CAD build for the part. Positions are in the model's coordinates, mm. Face numbers are marked on the shaded views. A direction names the side the tool comes from. Round coordinates to 2 decimals unless told otherwise and drop trailing zeros. Loops run counter-clockwise (first coordinate to the right, second up) from the corner with the lowest first, then second, coordinate; pieces in that order, holes last. Notation, with made-up numbers: M 33.5,86.5 L 62.5,86.5 A20 ccw 62.5,125.5 Z; hole C -8,-9.5 d9. An arc over 180 degrees is marked long. One line per item, written item: value. Start each with the question number.
from build123d import *


with BuildPart() as part:
    # Sketch1 → Revolve1 (revolve)
    with BuildSketch(Plane.XY):
        Polygon((0, 0), (-7.9629, 0), (-7.9629, -3.81), (-5.842, -5.334), (-5.842, -7.239), (-7.9629, -8.001), (-7.9629, -40.259), (-6.3754, -40.259), (-6.3754, -45.593), (-12.5, -45.593), (-12.5, -63.119), (-6.3754, -63.119), (-6.3754, -69.142247751), (-2.410616984, -74.041), (0, -74.041), align=None)
    revolve(axis=Axis((0, 0, 0), (0, 1, 0)))


solid = part.part
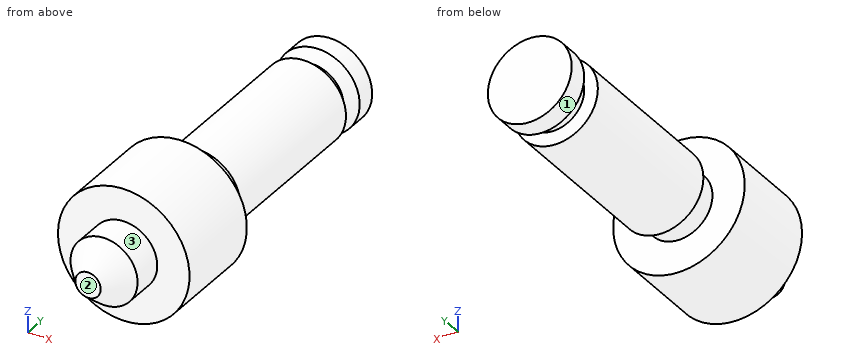
(1) Which spindle directions (+Z, -Z, +X, -X, +Y, -Y) get a long thin tool onto all of the face, cutting with end or side? Do the marked faces 1, 2 and 3. Say none if no direction does.
(2) Probe L1, parallel to Y at x = -6, z = -4; L2, parallel to Y at x = -2, z = -8.25; L3, parallel to Y at x = 6, z = 0.5. List the from-to ranges inside material, lowest first.
(3) Flat gauge pins, fed straight in: P1, Ø12, axis at x = 2.5, z = -8, coming from the -Y side; P2, Ø10, axis at x = 8, y = -17.5, coming from the -Z side; P3, Ø3, axis at x = -5.5, y = -60, coming from the +Z side; P4, Ø12, axis at x = -7, y = -8.5, coming from the +Z side. Where does each tip first touch, or does it go through?
(4) Slice it at C-C, the plane y = -67. List the corners of the cut face in (x, z), and give its area (3 significant figures).
(5) Slice it at B-B, the plane z = 0. List the corners of the cut face in (x, y).
(6) Slice it at D-D, the plane y = -50.5. List the corners of the cut face in (x, z), and give its area (3 significant figures).
(7) Slice it at A-A, the plane x = 0. List the corners of the cut face in (y, z), and give its area (3 significant figures).
Check result:
1. face 1: +Y
1. face 2: +Z, -Z, +X, -X, -Y
1. face 3: -Y
2. L1: y = -63.12 to -45.59, -40.26 to -7.73, -4.35 to 0
2. L2: y = -63.12 to -45.59
2. L3: y = -69.58 to -7.3, -5.21 to 0
3. P1: stops at y = -74.04
3. P2: stops at z = -7.38
3. P3: stops at z = 11.84
3. P4: stops at z = 7.9
4. outline: C 0,0 d12.75
4. area: 128 mm^2
5. outline: M -12.5,-63.12 L -6.38,-63.12 L -6.38,-69.14 L -2.41,-74.04 L 2.41,-74.04 L 6.38,-69.14 L 6.38,-63.12 L 12.5,-63.12 L 12.5,-45.59 L 6.38,-45.59 L 6.38,-40.26 L 7.96,-40.26 L 7.96,-8 L 5.84,-7.24 L 5.84,-5.33 L 7.96,-3.81 L 7.96,0 L -7.96,0 L -7.96,-3.81 L -5.84,-5.33 L -5.84,-7.24 L -7.96,-8 L -7.96,-40.26 L -6.38,-40.26 L -6.38,-45.59 L -12.5,-45.59 Z
6. outline: C 0,0 d25
6. area: 491 mm^2
7. outline: M -74.04,-2.41 L -69.14,-6.38 L -63.12,-6.38 L -63.12,-12.5 L -45.59,-12.5 L -45.59,-6.38 L -40.26,-6.38 L -40.26,-7.96 L -8,-7.96 L -7.24,-5.84 L -5.33,-5.84 L -3.81,-7.96 L 0,-7.96 L 0,7.96 L -3.81,7.96 L -5.33,5.84 L -7.24,5.84 L -8,7.96 L -40.26,7.96 L -40.26,6.38 L -45.59,6.38 L -45.59,12.5 L -63.12,12.5 L -63.12,6.38 L -69.14,6.38 L -74.04,2.41 Z
7. area: 1,250 mm^2
